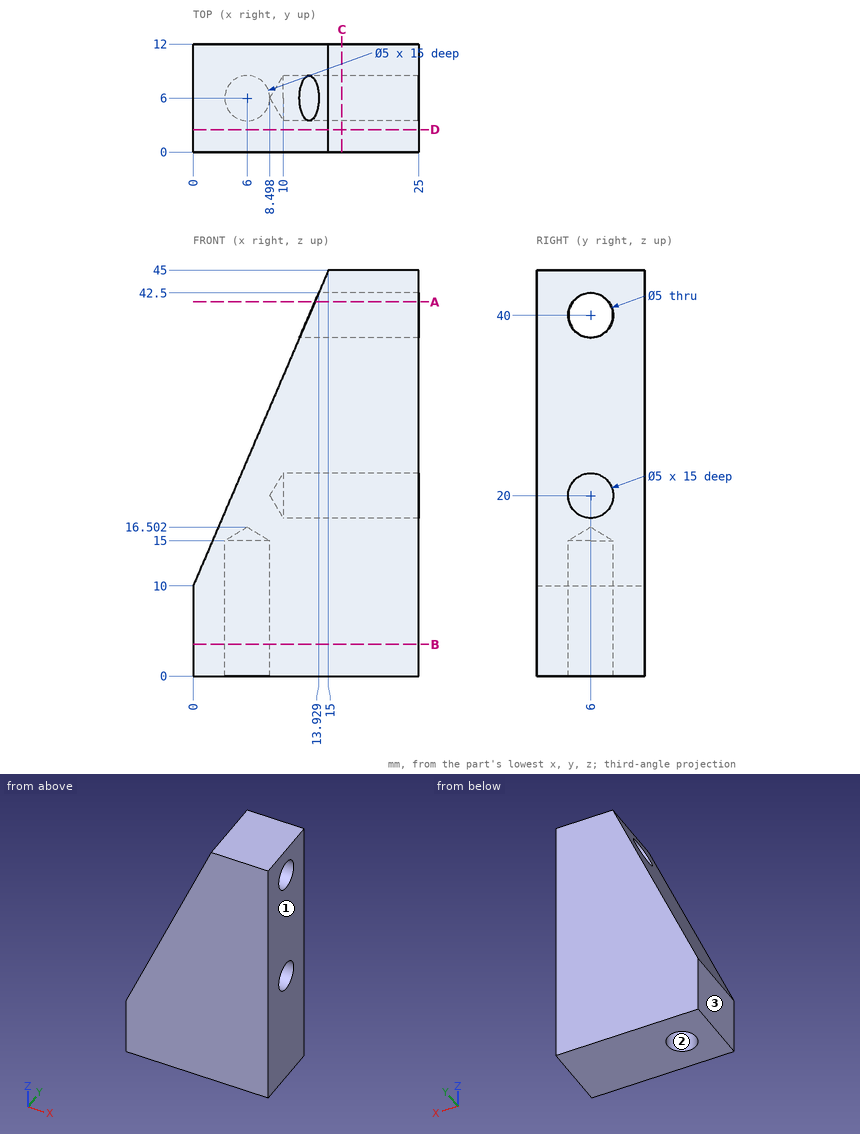
The drawing under review shows one solid part. Ordinate dimensions are in mm from its lowest x, y, z. Coordinates: 2 decimals unless noted, no trailing zeros. Loops run counter-clockwise (first coordinate to the right, second up) from the corner with the lowest first, then second, coordinate; pieces in that order, holes last.
Item 1: Add section B-B (z = 3.5). Write out the cut boundary in (x, y), and give its area (3 significant figures).
Completed:
outline: (0, 0) - (25, 0) - (25, 12) - (0, 12) - close; hole circle Ø5 at (6, 6)
area: 280 mm2
Item 2: Add section D-D (y = 2.5). Write out the cut boundary in (x, z).
Completed:
outline: (0, 0) - (25, 0) - (25, 45) - (15, 45) - (0, 10) - close
Item 3: Add section A-A (z = 41.5). Write out the cut boundary in (x, y).
Completed:
outline: (13.5, 0) - (25, 0) - (25, 4) - (13.5, 4) - close; (13.5, 8) - (25, 8) - (25, 12) - (13.5, 12) - close
Item 4: Draft analysis for pull direction X (two halves, no side actions). For the marked faces 1, 2 and 3, state which applies: pulls with the +X half, pulls with the -X half, needs draft (parallel to the pull), parting line crosses it, or undercut.
Completed:
face 1: pulls with the +X half
face 2: undercut
face 3: pulls with the -X half
Item 5: Add section C-C (x = 16.5). Write out the cut boundary in (y, z), and give its area (3 significant figures).
Completed:
outline: (0, 0) - (12, 0) - (12, 45) - (0, 45) - close; hole circle Ø5 at (6, 20); hole circle Ø5 at (6, 40)
area: 501 mm2
Item 6: Clearance check with flat-ended pins moving along their axes: pin 1 (3 mm diameter, centred on x = 6, y = 6, fed in from -Z); pin 2 (5 mm diameter, centred on x = 19.5, y = 8, fed in from -Z); pin 3 (6 mm diameter, centred on y = 6, z = 20, fed in from -X). State where each tip first meets the part, or that it passes through.
Completed:
pin 1: stops at z = 15.6
pin 2: stops at z = 0
pin 3: stops at x = 3
Item 7: Wall thickness on L1, parallel to Z at x = 20, y = 6; L2, parallel to X at y = 6, z = 4.5; L3, parallel to Y at x = 6, z = 11: over which ranges is each line inside the solid? List them lowest first.
Completed:
L1: z = 0 to 17.5, 22.5 to 37.5, 42.5 to 45
L2: x = 0 to 3.5, 8.5 to 25
L3: y = 0 to 3.5, 8.5 to 12
